```python
from build123d import *

# Parameters (mm, degrees)
F1_DEPTH     = 31
F2_R         = 18.8
F3_DEPTH     = 6
F4_R         = 5
F5_DEPTH     = 18
F6_R         = 4
F8_W         = 41
F8_H         = 41
F9_DEPTH     = 10
F10_T1_DEPTH = 20
F12_DEPTH    = 20
F13_W        = 41
F13_H        = 41
F14_DEPTH    = 10
F15_R        = 4


# Not quite as in the source:
# - a fillet or chamfer that OpenCascade refuses, or shapes differently, is made with other operations: its cross-section is extruded or revolved along the edge and cut away or added


with BuildPart() as f1:
    # F0 (on Top) → F1 (new body)
    with BuildSketch(Plane.XY):
        with BuildLine():
            Line((18.7383297014, 18.7383297014), (21, 21))
            Line((21, 21), (11.6189500386, 21))
            ThreePointArc((11.6189500386, 21), (13.4178535673, 19.8987739735), (15.1131239157, 18.6438591903))
            ThreePointArc((15.1131239157, 18.6438591903), (16.9054364798, 19.4697143183), (18.7383297014, 18.7383297014))
        make_face()
        with BuildLine():
            ThreePointArc((-15.1131239157, 18.6438591903), (-13.4178535673, 19.8987739735), (-11.6189500386, 21))
            Line((-11.6189500386, 21), (-21, 21))
            Line((-21, 21), (-18.7383297014, 18.7383297014))
            ThreePointArc((-18.7383297014, 18.7383297014), (-16.9054364798, 19.4697143183), (-15.1131239157, 18.6438591903))
        make_face()
        with BuildLine():
            Line((11.6189500386, -21), (21, -21))
            Line((21, -21), (18.7383297014, -18.7383297014))
            ThreePointArc((18.7383297014, -18.7383297014), (16.9054364798, -19.4697143183), (15.1131239157, -18.6438591903))
            ThreePointArc((15.1131239157, -18.6438591903), (13.4178535673, -19.8987739735), (11.6189500386, -21))
        make_face()
        with BuildLine():
            Line((-21, -21), (-11.6189500386, -21))
            ThreePointArc((-11.6189500386, -21), (-13.4178535673, -19.8987739735), (-15.1131239157, -18.6438591903))
            ThreePointArc((-15.1131239157, -18.6438591903), (-16.9054364798, -19.4697143183), (-18.7383297014, -18.7383297014))
            Line((-18.7383297014, -18.7383297014), (-21, -21))
        make_face()
        with BuildLine():
            Line((21, 11.6189500386), (21, 21))
            Line((21, 21), (18.7383297014, 18.7383297014))
            ThreePointArc((18.7383297014, 18.7383297014), (19.2802615798, 17.9272713294), (19.4705627485, 16.9705627485))
            ThreePointArc((19.4705627485, 16.9705627485), (19.2545549885, 15.954010021), (18.6438591903, 15.1131239157))
            ThreePointArc((18.6438591903, 15.1131239157), (19.8987739735, 13.4178535673), (21, 11.6189500386))
        make_face()
        with BuildLine():
            Line((21, -21), (21, -11.6189500386))
            ThreePointArc((21, -11.6189500386), (19.8987739735, -13.4178535673), (18.6438591903, -15.1131239157))
            ThreePointArc((18.6438591903, -15.1131239157), (19.2545549885, -15.954010021), (19.4705627485, -16.9705627485))
            ThreePointArc((19.4705627485, -16.9705627485), (19.2802615798, -17.9272713294), (18.7383297014, -18.7383297014))
            Line((18.7383297014, -18.7383297014), (21, -21))
        make_face()
        with BuildLine():
            Line((-18.7383297014, 18.7383297014), (-21, 21))
            Line((-21, 21), (-21, 11.6189500386))
            ThreePointArc((-21, 11.6189500386), (-19.8987739735, 13.4178535673), (-18.6438591903, 15.1131239157))
            ThreePointArc((-18.6438591903, 15.1131239157), (-19.4697143183, 16.9054364798), (-18.7383297014, 18.7383297014))
        make_face()
        with BuildLine():
            ThreePointArc((-18.6438591903, -15.1131239157), (-19.8987739735, -13.4178535673), (-21, -11.6189500386))
            Line((-21, -11.6189500386), (-21, -21))
            Line((-21, -21), (-18.7383297014, -18.7383297014))
            ThreePointArc((-18.7383297014, -18.7383297014), (-19.4697143183, -16.9054364798), (-18.6438591903, -15.1131239157))
        make_face()
        with BuildLine():
            ThreePointArc((15.1131239157, 18.6438591903), (13.4178535673, 19.8987739735), (11.6189500386, 21))
            Line((11.6189500386, 21), (-11.6189500386, 21))
            ThreePointArc((-11.6189500386, 21), (-13.4178535673, 19.8987739735), (-15.1131239157, 18.6438591903))
            ThreePointArc((-15.1131239157, 18.6438591903), (-14.6367250204, 17.8667778225), (-14.4705627485, 16.9705627485))
            ThreePointArc((-14.4705627485, 16.9705627485), (-14.6608639172, 16.0138541676), (-15.2027957955, 15.2027957955))
            Line((-15.2027957955, 15.2027957955), (0, 0))
            Line((0, 0), (15.2027957955, 15.2027957955))
            ThreePointArc((15.2027957955, 15.2027957955), (14.4714111786, 16.9054364798), (15.1131239157, 18.6438591903))
        make_face()
        with BuildLine():
            Line((15.2027957955, -15.2027957955), (0, 0))
            Line((0, 0), (-15.2027957955, -15.2027957955))
            ThreePointArc((-15.2027957955, -15.2027957955), (-14.6608639172, -16.0138541676), (-14.4705627485, -16.9705627485))
            ThreePointArc((-14.4705627485, -16.9705627485), (-14.6367250204, -17.8667778225), (-15.1131239157, -18.6438591903))
            ThreePointArc((-15.1131239157, -18.6438591903), (-13.4178535673, -19.8987739735), (-11.6189500386, -21))
            Line((-11.6189500386, -21), (11.6189500386, -21))
            ThreePointArc((11.6189500386, -21), (13.4178535673, -19.8987739735), (15.1131239157, -18.6438591903))
            ThreePointArc((15.1131239157, -18.6438591903), (14.4714111786, -16.9054364798), (15.2027957955, -15.2027957955))
        make_face()
        with BuildLine():
            Line((21, -11.6189500386), (21, 11.6189500386))
            ThreePointArc((21, 11.6189500386), (19.8987739735, 13.4178535673), (18.6438591903, 15.1131239157))
            ThreePointArc((18.6438591903, 15.1131239157), (16.9054364798, 14.4714111786), (15.2027957955, 15.2027957955))
            Line((15.2027957955, 15.2027957955), (0, 0))
            Line((0, 0), (15.2027957955, -15.2027957955))
            ThreePointArc((15.2027957955, -15.2027957955), (16.9054364798, -14.4714111786), (18.6438591903, -15.1131239157))
            ThreePointArc((18.6438591903, -15.1131239157), (19.8987739735, -13.4178535673), (21, -11.6189500386))
        make_face()
        with BuildLine():
            ThreePointArc((-18.6438591903, 15.1131239157), (-19.8987739735, 13.4178535673), (-21, 11.6189500386))
            Line((-21, 11.6189500386), (-21, -11.6189500386))
            ThreePointArc((-21, -11.6189500386), (-19.8987739735, -13.4178535673), (-18.6438591903, -15.1131239157))
            ThreePointArc((-18.6438591903, -15.1131239157), (-16.9054364798, -14.4714111786), (-15.2027957955, -15.2027957955))
            Line((-15.2027957955, -15.2027957955), (0, 0))
            Line((0, 0), (-15.2027957955, 15.2027957955))
            ThreePointArc((-15.2027957955, 15.2027957955), (-16.9054364798, 14.4714111786), (-18.6438591903, 15.1131239157))
        make_face()
    extrude(amount=F1_DEPTH)

    # F2 (on face) → F3 (join)
    with BuildSketch(Plane.XY.offset(31)):
        Circle(F2_R)
    extrude(amount=F3_DEPTH)

    # F4 (on face) → F5 (join)
    with BuildSketch(Plane.XY.offset(37)):
        Circle(F4_R)
    extrude(amount=F5_DEPTH)

    # F6
    f6_edges = [f1.edges().sort_by_distance(p)[0] for p in [
        (-21, -21, 15.5),
        (-21, 21, 15.5),
        (21, 21, 15.5),
        (21, -21, 15.5),
    ]]
    fillet(f6_edges, radius=F6_R)

    # F8 (on face) → F9 (join)
    with BuildSketch(Plane(origin=(0, 0, 0), x_dir=(1, 0, 0), z_dir=(0, 0, -1))):
        Rectangle(F8_W, F8_H)
    extrude(amount=F9_DEPTH)

    # F10: fillet of radius 4 on 4 edges, made by hand

    # F10_s2 → F10_t1 (cut)
    with BuildSketch(Plane.XY.offset(-20)):
        with BuildLine():
            ThreePointArc((20.5, -16.5), (19.3284271247, -19.3284271247), (16.5, -20.5))
            Line((16.5, -20.5), (20.5, -20.5))
            Line((20.5, -20.5), (20.5, -16.5))
        make_face()
        with BuildLine():
            ThreePointArc((16.5, 20.5), (19.3284271247, 19.3284271247), (20.5, 16.5))
            Line((20.5, 16.5), (20.5, 20.5))
            Line((20.5, 20.5), (16.5, 20.5))
        make_face()
        with BuildLine():
            ThreePointArc((-16.5, 20.5), (-19.3284271247, 19.3284271247), (-20.5, 16.5))
            Line((-20.5, 16.5), (-20.5, 20.5))
            Line((-20.5, 20.5), (-16.5, 20.5))
        make_face()
        with BuildLine():
            ThreePointArc((-20.5, -16.5), (-19.3284271247, -19.3284271247), (-16.5, -20.5))
            Line((-16.5, -20.5), (-20.5, -20.5))
            Line((-20.5, -20.5), (-20.5, -16.5))
        make_face()
    extrude(amount=F10_T1_DEPTH, mode=Mode.SUBTRACT)

    # F11 (on face) → F12 (join)
    with BuildSketch(Plane(origin=(0, 0, -10), x_dir=(1, 0, 0), z_dir=(0, 0, -1))):
        Polygon((-15.5, 20.5), (-20.5, 15.5), (-15.5, 15.5), align=None)
        Polygon((15.5, 15.5), (20.5, 15.5), (15.5, 20.5), align=None)
        Polygon((15.5, -15.5), (15.5, -20.5), (20.5, -15.5), align=None)
        Polygon((-20.5, -15.5), (-15.5, -20.5), (-15.5, -15.5), align=None)
        Polygon((-15.5, -20.5), (15.5, -20.5), (15.5, -15.5), (20.5, -15.5), (20.5, 15.5), (15.5, 15.5), (15.5, 20.5), (-15.5, 20.5), (-15.5, 15.5), (-20.5, 15.5), (-20.5, -15.5), (-15.5, -15.5), align=None)
    extrude(amount=F12_DEPTH)

    # F13 (on face) → F14 (join)
    with BuildSketch(Plane(origin=(0, 0, -30), x_dir=(1, 0, 0), z_dir=(0, 0, -1))):
        Rectangle(F13_W, F13_H)
    extrude(amount=F14_DEPTH)

    # F15
    f15_edges = [f1.edges().sort_by_distance(p)[0] for p in [
        (20.5, -20.5, -35),
        (-20.5, -20.5, -35),
        (20.5, 20.5, -35),
        (-20.5, 20.5, -35),
    ]]
    fillet(f15_edges, radius=F15_R)


solid = f1.part
```
The listing builds one solid part. Answer for the finished solid, in the listing's coordinates (mm). A direction names the side the tool comes from. Coordinates: 2 decimals unless noted, no trailing zeros. Loops run counter-clockwise (first coordinate to the right, second up) from the corner with the lowest first, then second, coordinate; pieces in that order, holes last. Notation, with made-up numbers: M -31.75,83.25 L 6.25,83.25 A24 ccw 6.25,101.25 Z; hole C -31,-10.75 d9. An arc over 180 degrees is marked long. Answer as a JSON object with one key per item and string values. Group by question number.
Item 1: Section D-D (x = -6.5) is taken. Write down the section's boundary in (y, z).
Item 2: Consider L1, parallel to Y at x = 18.5, z = 21; L2, parallel to Z at x = -8.5, y = 16; L3, parallel to Y at x = 11, z = -28. Determine where each line is inside the solid, lowest interval first.
Item 3: Which of the six approach directions +Z, -Z, +X, -X, +Y, -Y give full straight-line access (tool end or side, diameter ignored) to faces 1 (the face through (17, -17, 0)), 2 (the face through (19, -19, -30)), 3 (the face through (-19.297, 19.359, -5.07)), 4 (the face through (20.5, 0, -20))?
Item 4: Each of these flat-tipped pins is pushed along its axis until it touches: P1, Ø16.5, axis at y = -3, z = -13.5, coming from the -X side; P2, Ø1.5, axis at x = 17, y = 19, coming from the +Z side; P3, Ø2.5, axis at x = -17, y = 18, coming from the +Z side. Where does it stop, or does it pass through?
Item 5: Section A-A (z = 25) is taken. Write down the section's boundary in (x, y), and give its area (3 significant figures).
Item 6: Section B-B (x = 0) is taken. Write down the section's boundary in (y, z).
Item 7: Determine the mould class of faces 5 (the face through (-17, -17, 0)), 6 (the face through (19.797, 19.859, 15.717)), 7 (the face through (19, -19, -10)) for opening direction Z: +Z half, -Z half, draft (parallel to the pull), parting line (faces both ways), or undercut.
Solved:
{
 "1": {"outline": "M -21,0 L -20.5,0 L -20.5,-40 L 20.5,-40 L 20.5,0 L 21,0 L 21,31 L 17.64,31 L 17.64,37 L -17.64,37 L -17.64,31 L -21,31 Z"},
 "2": {"L1": "y = -20.71 to -18.95, -14.99 to 14.99, 18.95 to 20.71", "L2": "z = -40 to 37", "L3": "y = -20.5 to 20.5"},
 "3": {"face 1": "+Z", "face 2": "+X, -Y", "face 3": "-Z, -X, +Y", "face 4": "-Z, +X, +Y, -Y"},
 "4": {"P1": "stops at x = -20.5", "P2": "stops at z = 31", "P3": "stops at z = 0"},
 "5": {"outline": "M -21,-17 A4 ccw -17,-21 L 17,-21 A4 ccw 21,-17 L 21,17 A4 ccw 17,21 L -17,21 A4 ccw -21,17 Z; hole C -16.97,-16.97 d5; hole C -16.97,16.97 d5; hole C 16.97,-16.97 d5; hole C 16.97,16.97 d5", "area": "1,670 mm2"},
 "6": {"outline": "M -21,0 L -20.5,0 L -20.5,-40 L 20.5,-40 L 20.5,0 L 21,0 L 21,31 L 18.8,31 L 18.8,37 L 5,37 L 5,55 L -5,55 L -5,37 L -18.8,37 L -18.8,31 L -21,31 Z"},
 "7": {"face 5": "+Z half", "face 6": "draft", "face 7": "undercut"}
}
